```python
from build123d import *

# Parameters (mm, degrees)
CHAMFER_1_SIZE = 0.5
CHAMFER_2_SIZE = 1


with BuildPart() as part:
    # 스케치2 → 회전1 (revolve)
    with BuildSketch(Plane(origin=(0, 0, 0), x_dir=(0, 0, -1), z_dir=(1, 0, 0)), mode=Mode.PRIVATE) as revolve_1_sk:
        Polygon((3, 0), (10, 0), (10, -2), (8, -2), (8, -3.5), (10, -5.5), (10, -7), (7.4, -7), (7.4, -10), (7.9, -10.5), (7.9, -13), (7.4, -13.5), (7.4, -15), (5.9, -15), (5.9, -16.5), (3, -16.5), align=None)
    revolve(revolve_1_sk.sketch.rotate(Axis((0, 0, 0), (0, -1, 0)), 180), axis=Axis((0, 0, 0), (0, -1, 0)))

    # 모따기1
    chamfer_1_edges = [part.edges().sort_by_distance(p)[0] for p in [
        (0, 0, -10),
        (0, -16.5, -5.9),
    ]]
    chamfer(chamfer_1_edges, length=CHAMFER_1_SIZE)

    # 모따기2
    chamfer_2_edges = [part.edges().sort_by_distance(p)[0] for p in [
        (0, 0, -3),
    ]]
    chamfer(chamfer_2_edges, length=CHAMFER_2_SIZE)


solid = part.part
```
Source: CAD feature listing. Evaluate the final solid. Frame: model axes, mm. A direction names the side the tool comes from. Give positions to 0.01 mm unless a question says otherwise; leave off trailing zeros. Loops run counter-clockwise (first coordinate to the right, second up) from the corner with the lowest first, then second, coordinate; pieces in that order, holes last. Notation, with made-up numbers: (-12.75, -38.75) -> (39.25, -38.75) arc R35 cw to (39.25, -2.75) -> close; hole circle Ø11 at (16, 32). An arc over 180 degrees is marked (long way). Use a Markdown table: item, result. Add a question column.
(1) Ray query, line 1 (X direction, y = -5, z = 0); line 2 (X direction, y = -6, z = 0); line 3 (Z direction, x = -0.5, y = -10.25). Return the intervals inside material, ascending.
(2) Section query A-A (y = -8). Output: boundary loops of the cut face in (x, z), then the cut area to 3 significant figures.
(3) Section query B-B (y = -1.5). Output: boundary loops of the cut face in (x, z).
(4) Pull-direction query (X, two-part tool) for faces 1 (the face through (7.224, -14.26, -1.604)), 2 (the face through (-0.9, -8.64, 2.86)), 3 (the face through (-7.5, -7, 1.4)); classes: +X half, -X half, draft (parallel to the pull), parting line (faces both ways), or undercut.
(5) Access query for faces 4 (the face through (-8.2, -2, 0)), 5 (the face through (2, -15, -6)), 6 (the face through (0, -6, -10)). Directions: +Z, -Z, +X, -X, +Y, -Y. A direction counts if a zero-diameter tool reaches every point of the face in a straight line with its end or side. Return the directions, or none.
(6) First-contact query: pin 1 Ø3 at (y, z) = (-2.5, 6) entering from -X; pin 2 Ø6 at (x, z) = (6, -7.5) entering from -Y; pin 3 Ø5 at (y, z) = (-5.5, -6.5) entering from -X. Flat tips, straight axial feed; report the tip coordinate or a pass-through.
Checked values:
| question | item | result |
|---|---|---|
| 1 | line 1 | -9.5 to -3, 3 to 9.5 |
| 1 | line 2 | -10 to -3, 3 to 10 |
| 1 | line 3 | -7.63 to -2.96, 2.96 to 7.63 |
| 2 | outline | circle Ø14.8 at (0, 0); hole circle Ø6 at (0, 0) |
| 2 | area | 144 mm^2 |
| 3 | outline | circle Ø20 at (0, 0); hole circle Ø6 at (0, 0) |
| 4 | face 1 | parting line |
| 4 | face 2 | undercut |
| 4 | face 3 | draft |
| 5 | face 4 | none |
| 5 | face 5 | -Y |
| 5 | face 6 | +Y, -Y |
| 6 | pin 1 | x = -8.89 |
| 6 | pin 2 | y = -15 |
| 6 | pin 3 | x = -9.17 |
